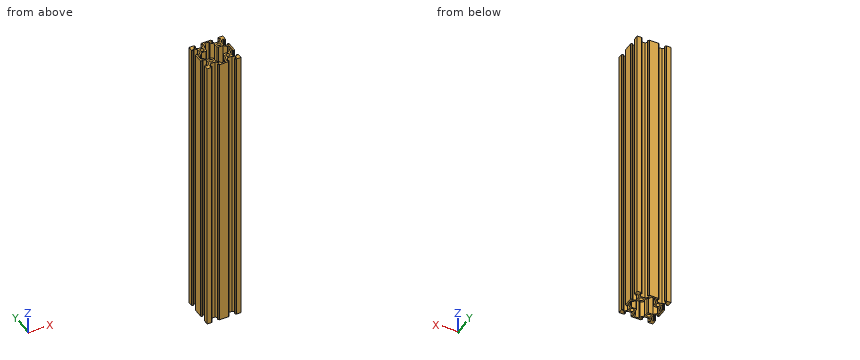
from build123d import *

# Parameters (mm, degrees)
SKETCH1_W           = 40
SKETCH1_H           = 40
BOSS_EXTRUDE1_DEPTH = 345
SKETCH2_R           = 2.3
CUT_EXTRUDE1_DEPTH  = 345
CUT_EXTRUDE2_DEPTH  = 345


with BuildPart() as part:
    # Sketch1 → Boss-Extrude1 (new body)
    with BuildSketch(Plane.XY):
        with Locations((20, 20)):
            Rectangle(SKETCH1_W, SKETCH1_H)
    extrude(amount=-BOSS_EXTRUDE1_DEPTH)

    # Sketch2 → Cut-Extrude1 (cut)
    with BuildSketch(Plane.XY):
        with Locations((10, 30)):
            Circle(SKETCH2_R)
        with Locations((30, 30)):
            Circle(SKETCH2_R)
        with Locations((30, 10)):
            Circle(SKETCH2_R)
        with Locations((10, 10)):
            Circle(SKETCH2_R)
        Polygon((6.605, 38.815), (6.605, 38.2), (4.5, 38.2), (4.5, 36.772792206), (7.372792206, 33.9), (12.627207794, 33.9), (15.5, 36.772792206), (15.5, 38.2), (13.395, 38.2), (13.395, 38.815), (14.58, 40), (5.42, 40), align=None)
        Polygon((26.605, 38.815), (25.42, 40), (34.58, 40), (33.395, 38.815), (33.395, 38.2), (35.5, 38.2), (35.5, 36.772792206), (32.627207794, 33.9), (27.372792206, 33.9), (24.5, 36.772792206), (24.5, 38.2), (26.605, 38.2), align=None)
        Polygon((26.605, 1.8), (26.605, 1.185), (25.42, 0), (34.58, 0), (33.395, 1.185), (33.395, 1.8), (35.5, 1.8), (35.5, 3.227207794), (32.627207794, 6.1), (27.372792206, 6.1), (24.5, 3.227207794), (24.5, 1.8), align=None)
        Polygon((13.395, 1.185), (14.58, 0), (5.42, 0), (6.605, 1.185), (6.605, 1.8), (4.5, 1.8), (4.5, 3.227207794), (7.372792206, 6.1), (12.627207794, 6.1), (15.5, 3.227207794), (15.5, 1.8), (13.395, 1.8), align=None)
        Polygon((1.8, 13.395), (1.185, 13.395), (0, 14.58), (0, 5.42), (1.185, 6.605), (1.8, 6.605), (1.8, 4.5), (3.227207794, 4.5), (6.1, 7.372792206), (6.1, 12.627207794), (3.227207794, 15.5), (1.8, 15.5), align=None)
        Polygon((1.185, 26.605), (0, 25.42), (0, 34.58), (1.185, 33.395), (1.8, 33.395), (1.8, 35.5), (3.227207794, 35.5), (6.1, 32.627207794), (6.1, 27.372792206), (3.227207794, 24.5), (1.8, 24.5), (1.8, 26.605), align=None)
        Polygon((38.2, 15.5), (38.2, 13.395), (38.815, 13.395), (40, 14.58), (40, 5.42), (38.815, 6.605), (38.2, 6.605), (38.2, 4.5), (36.772792206, 4.5), (33.9, 7.372792206), (33.9, 12.627207794), (36.772792206, 15.5), align=None)
        Polygon((38.2, 26.605), (38.815, 26.605), (40, 25.42), (40, 34.58), (38.815, 33.395), (38.2, 33.395), (38.2, 35.5), (36.772792206, 35.5), (33.9, 32.627207794), (33.9, 27.372792206), (36.772792206, 24.5), (38.2, 24.5), align=None)
    extrude(amount=-CUT_EXTRUDE1_DEPTH, mode=Mode.SUBTRACT)

    # Sketch3 → Cut-Extrude2 (cut)
    with BuildSketch(Plane.XY):
        Polygon((17.3, 38.2), (22.7, 38.2), (22.7, 36.027207794), (26.1, 32.627207794), (26.1, 27.372792206), (27.372792206, 26.1), (32.627207794, 26.1), (36.027207794, 22.7), (38.2, 22.7), (38.2, 17.3), (36.027207794, 17.3), (32.627207794, 13.9), (27.372792206, 13.9), (26.1, 12.627207794), (26.1, 7.372792206), (22.7, 3.972792206), (22.7, 1.8), (17.3, 1.8), (17.3, 3.972792206), (13.9, 7.372792206), (13.9, 12.627207794), (12.627207794, 13.9), (7.372792206, 13.9), (3.972792206, 17.3), (1.8, 17.3), (1.8, 22.7), (3.972792206, 22.7), (7.372792206, 26.1), (12.627207794, 26.1), (13.9, 27.372792206), (13.9, 32.627207794), (17.3, 36.027207794), align=None)
    extrude(amount=-CUT_EXTRUDE2_DEPTH, mode=Mode.SUBTRACT)


solid = part.part
The listing builds one solid part. Answer for the finished solid, in the listing's coordinates (mm). Give positions to 0.01 mm unless a question says otherwise; leave off trailing zeros.
1) Section A-A (z = -117) is taken. Count the separate pieces of the cut face and the enclosed holes in it, and give its area (3 significant figures).
2) Given P1, Ø10, axis at x = 29, y = 5, coming from the -Z side; P2, Ø1.6, axis at y = 11, z = -106.5, coming from the -X side; P3, Ø2.5, axis at y = 30, z = -87, coming from the +X side; P4, Ø5, axis at y = 9, z = -48.5, coming from the +X side, each flat-ended and moving along its own axis, determine where each tip first touches the part or whether it passes through.
3) Find the intervals of material crossed by L1, parallel to Y at x = 30, z = -129; L2, parallel to Y at x = 38.5, z = -50.5 (3 decimals); L3, parallel to Y at x = 26, z = -72.5, in increasing order.
Response:
1. separate pieces: 1
1. enclosed holes: 5
1. area: 475 mm2
2. P1: stops at z = -345
2. P2: stops at x = 6.1
2. P3: stops at x = 33.9
2. P4: stops at x = 38.92
3. L1: y = 6.1 to 7.7, 12.3 to 13.9, 26.1 to 27.7, 32.3 to 33.9
3. L2: y = 0 to 6.605, 13.395 to 26.605, 33.395 to 40
3. L3: y = 0.58 to 1.8, 4.73 to 7.27, 32.73 to 35.27, 38.2 to 39.42
